from build123d import *

# Parameters (mm, degrees)
SKETCH009_R     = 21
PAD002_DEPTH    = 6
SKETCH010_R     = 4
PAD003_DEPTH    = 6
SKETCH011_R     = 1.65
SKETCH011_R_2   = 1.9
POCKET007_DEPTH = 6.001
SKETCH012_R     = 9.05
POCKET008_DEPTH = 4
SKETCH013_R     = 8.05
POCKET009_DEPTH = 6.001


with BuildPart() as part:
    # Sketch009 → Pad002 (new body)
    with BuildSketch(Plane.XY):
        Circle(SKETCH009_R)
    extrude(amount=PAD002_DEPTH)

    # Sketch010 (on DatumPlane) → Pad003 (join)
    with BuildSketch(Plane.XY.offset(6)):
        with Locations((-12.727922, 12.727922)):
            Circle(SKETCH010_R)
        with Locations((0, 18)):
            Circle(SKETCH010_R)
        with Locations((12.727922, 12.727922)):
            Circle(SKETCH010_R)
        with Locations((15.588457, -9)):
            Circle(SKETCH010_R)
        with Locations((-15.588457, -9)):
            Circle(SKETCH010_R)
    extrude(amount=-PAD003_DEPTH)

    # Sketch011 (on DatumPlane) → Pocket007 (cut, through all)
    with BuildSketch(Plane.XY.offset(6)):
        with Locations((-12.727922, 12.727922)):
            Circle(SKETCH011_R)
        with Locations((0, 18)):
            Circle(SKETCH011_R_2)
        with Locations((12.727922, 12.727922)):
            Circle(SKETCH011_R)
        with Locations((-15.588457, -9)):
            Circle(SKETCH011_R_2)
        with Locations((15.588457, -9)):
            Circle(SKETCH011_R_2)
    extrude(amount=-POCKET007_DEPTH, mode=Mode.SUBTRACT)

    # Sketch012 (on DatumPlane) → Pocket008 (cut)
    with BuildSketch(Plane.XY.offset(6)):
        Circle(SKETCH012_R)
    extrude(amount=-POCKET008_DEPTH, mode=Mode.SUBTRACT)

    # Sketch013 (on DatumPlane) → Pocket009 (cut, through all)
    with BuildSketch(Plane.XY.offset(6)):
        Circle(SKETCH013_R)
    extrude(amount=-POCKET009_DEPTH, mode=Mode.SUBTRACT)


with BuildPart() as part_1:
    # Body001 placement: moved
    add(part.part.moved(Location((0, 0, 14))))


solid = part_1.part
Source: CAD feature listing. Evaluate the final solid. Frame: model axes, mm. A direction names the side the tool comes from. Coordinates: 2 decimals unless noted, no trailing zeros. Loops run counter-clockwise (first coordinate to the right, second up) from the corner with the lowest first, then second, coordinate; pieces in that order, holes last. Notation, with made-up numbers: (-4, 22) -> (9, 22) arc R22 cw to (9, 49) -> close; hole circle Ø5 at (31.5, -2.5). An arc over 180 degrees is marked (long way). Answer in a Markdown table with one row per item. Add a question column.
Q1. Section D-D on z = 14.8. Return the cut outline in (x, y), and give its area (3 significant figures).
Q2. Section A-A on y = 0. Return the cut outline in (x, z), and give its area (3 significant figures).
Q3. Pull-direction query (X, two-part tool) for faces 3 (the face through (-20.8, 2.9, 17)), 4 (the face through (-10, 1, 20)), 5 (the face through (17.344, -9.728, 17.042)), 6 (the face through (-0.247, 19.884, 17.042)); classes: pulls with the +X half, pulls with the -X half, needs draft (parallel to the pull), parting line crosses it, or undercut.
Q4. Section B-B on x = 0. Return the cut outline in (y, z).
Q5. Reachability of faces 1 (the face through (8.63, 2.72, 18.03)), 2 (the face through (-14.376, 12.8, 17.042)) from +Z, -Z, +X, -X, +Y, -Y: full face, straight path, thin tool, end or side. Return the list, or none.
Q6. Ray query, line 1 along Y through (x, z) = (0, 15.2); line 2 along Y through (x, z) = (0, 17.7); line 3 along X through (y, z) = (12, 14.35). Return the intervals inside material, ascending.
Q7. Contact query for flat-ended pins moving along their axis: pin 1 Ø1 at (x, z) = (-10.5, 17.5) entering from -Y; pin 2 Ø2.5 at (x, y) = (-12.73, 12.73) entering from +Z; pin 3 Ø9 at (x, y) = (0, 4.5) entering from +Z; pin 4 Ø3 at (y, z) = (14, 15.5) entering from -X. Output: stop coordinate, or through.
Q8. Section C-C on x = 16. Return the cut outline in (y, z), and give its area (3 significant figures).
Computed values:
| question | item | result |
|---|---|---|
| 1 | outline | (-19.44, -7.93) arc R4 ccw to (-16.59, -12.87) arc R21 ccw to (16.59, -12.87) arc R4 ccw to (19.44, -7.93) arc R21 ccw to (16.73, 12.7) arc R4 ccw to (12.7, 16.73) arc R21 ccw to (2.85, 20.81) arc R4 ccw to (-2.85, 20.81) arc R21 ccw to (-12.7, 16.73) arc R4 ccw to (-16.73, 12.7) arc R21 ccw to start; hole circle Ø3.8 at (-15.59, -9); hole circle Ø3.3 at (-12.73, 12.73); hole circle Ø16.1 at (0, 0); hole circle Ø3.8 at (0, 18); hole circle Ø3.3 at (12.73, 12.73); hole circle Ø3.8 at (15.59, -9) |
| 1 | area | 1,150 mm^2 |
| 2 | outline | (-21, 14) -> (-8.05, 14) -> (-8.05, 16) -> (-9.05, 16) -> (-9.05, 20) -> (-21, 20) -> close; (8.05, 14) -> (21, 14) -> (21, 20) -> (9.05, 20) -> (9.05, 16) -> (8.05, 16) -> close |
| 2 | area | 147 mm^2 |
| 3 | face 3 | pulls with the -X half |
| 3 | face 4 | needs draft |
| 3 | face 5 | undercut |
| 3 | face 6 | undercut |
| 4 | outline | (-21, 14) -> (-8.05, 14) -> (-8.05, 16) -> (-9.05, 16) -> (-9.05, 20) -> (-21, 20) -> close; (8.05, 14) -> (16.1, 14) -> (16.1, 20) -> (9.05, 20) -> (9.05, 16) -> (8.05, 16) -> close; (19.9, 14) -> (22, 14) -> (22, 20) -> (19.9, 20) -> close |
| 5 | face 1 | +Z |
| 5 | face 2 | +Z, -Z |
| 6 | line 1 | y = -21 to -8.05, 8.05 to 16.1, 19.9 to 22 |
| 6 | line 2 | y = -21 to -9.05, 9.05 to 16.1, 19.9 to 22 |
| 6 | line 3 | x = -17.23 to -14.21, -11.25 to 11.25, 14.21 to 17.23 |
| 7 | pin 1 | stops at y = -18.47 |
| 7 | pin 2 | passes through |
| 7 | pin 3 | stops at z = 16 |
| 7 | pin 4 | stops at x = -16.87 |
| 8 | outline | (-13.6, 14) -> (-10.85, 14) -> (-10.85, 20) -> (-13.6, 20) -> close; (-7.15, 14) -> (15.03, 14) -> (15.03, 20) -> (-7.15, 20) -> close |
| 8 | area | 150 mm^2 |
